Source: CAD feature listing. Evaluate the final solid. Frame: model axes, mm. Face numbers are marked on the shaded views. A direction names the side the tool comes from. Give positions to 0.01 mm unless a question says otherwise; leave off trailing zeros. Loops run counter-clockwise (first coordinate to the right, second up) from the corner with the lowest first, then second, coordinate; pieces in that order, holes last. Notation, with made-up numbers: (60, 32) -> (100, 32) arc R8 cw to (100, 46) -> close; hole circle Ø5 at (-27, -0.75). An arc over 180 degrees is marked (long way). Answer as a JSON object with one key per item and string values. Group by question number.
from build123d import *

# Parameters (mm, degrees)
SKETCH1_W           = 40
SKETCH1_H           = 40
SKETCH1_R           = 2
BOSS_EXTRUDE1_DEPTH = 1
SKETCH2_W           = 40
SKETCH2_H           = 1
BOSS_EXTRUDE2_DEPTH = 46
CUT_EXTRUDE1_DEPTH  = 46


with BuildPart() as part:
    # Sketch1 → Boss-Extrude1 (new body)
    with BuildSketch(Plane(origin=(0, 0, 0), x_dir=(1, 0, 0), z_dir=(0, 1, 0))):
        Rectangle(SKETCH1_W, SKETCH1_H)
        with Locations(Location((-15, -12, 0), (0, 0, 270))):
            Circle(SKETCH1_R, mode=Mode.SUBTRACT)
        with Locations(Location((15, -12, 0), (0, 0, 270))):
            Circle(SKETCH1_R, mode=Mode.SUBTRACT)
        with Locations(Location((15, 12, 0), (0, 0, 270))):
            Circle(SKETCH1_R, mode=Mode.SUBTRACT)
        with Locations(Location((-15, 12, 0), (0, 0, 270))):
            Circle(SKETCH1_R, mode=Mode.SUBTRACT)
    extrude(amount=BOSS_EXTRUDE1_DEPTH)

    # Sketch2 → Boss-Extrude2 (add)
    with BuildSketch(Plane(origin=(0, 1, 0), x_dir=(1, 0, 0), z_dir=(0, 1, 0))):
        with Locations((0, 19.5)):
            Rectangle(SKETCH2_W, SKETCH2_H)
    extrude(amount=BOSS_EXTRUDE2_DEPTH)

    # Sketch3 → Cut-Extrude1 (cut)
    with BuildSketch(Plane.XY.offset(-19)):
        with BuildLine():
            Line((6, 19), (6, 35))
            ThreePointArc((6, 35), (0, 41), (-6, 35))
            Line((-6, 35), (-6, 19))
            ThreePointArc((-6, 19), (0, 13), (6, 19))
        make_face()
        with BuildLine():
            Line((-20, 47), (-20, 27))
            ThreePointArc((-20, 27), (-14.142135559, 41.142135688), (1.83e-07, 47))
            Line((1.83e-07, 47), (-20, 47))
        make_face()
        with BuildLine():
            ThreePointArc((1.83e-07, 47), (14.142135688, 41.142135559), (20, 27))
            Line((20, 27), (20, 47))
            Line((20, 47), (1.83e-07, 47))
        make_face()
    extrude(amount=-CUT_EXTRUDE1_DEPTH, mode=Mode.SUBTRACT)


solid = part.part
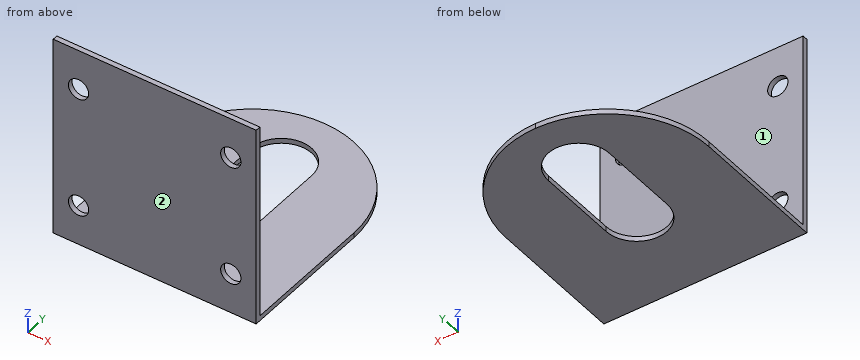
(1) Section query B-B on z = 12. Return the cut outline in (x, y), plus the area to 3 significant figures.
(2) Section query C-C on x = 15. Return the cut outline in (y, z), plus the area to 3 significant figures.
(3) First-contact query: pin 1 (3 mm diameter, centred on x = -15, z = 12, fed in from +Y); pin 2 (2 mm diameter, centred on x = -3, y = 7.5, fed in from +Z); pin 3 (19.5 mm diameter, centred on x = 0, z = -6, fed in from +Y); pin 4 (0.8 mm diameter, centred on y = 30, z = -19.5, fed in from +X). Flat tips, straight axial feed; report the tip coordinate or a pass-through.
(4) Section query A-A on y = 22. Return the cut outline in (x, z).
(5) Section query D-D on z = -6. Return the cut outline in (x, y).
(6) Access query for the marked faces 1 and 2. Directions: +Z, -Z, +X, -X, +Y, -Y. A direction counts if a zero-diameter tool reaches every point of the face in a straight line with its end or side. Return the directions, or none.
(7) Material intervals for line 1 (X direction, y = 0.5, z = 12); line 2 (Y direction, x = 6.5, z = 18); line 3 (Z direction, x = -2.5, y = 11.5), sorted ascending. Write a range as from..to.
Result:
{
 "1": {"outline": "(-20, 0) -> (-17, 0) -> (-17, 1) -> (-20, 1) -> close; (-13, 0) -> (13, 0) -> (13, 1) -> (-13, 1) -> close; (17, 0) -> (20, 0) -> (20, 1) -> (17, 1) -> close", "area": "32.0 mm²"},
 "2": {"outline": "(0, -20) -> (40.23, -20) -> (40.23, -19) -> (1, -19) -> (1, -14) -> (0, -14) -> close; (0, -10) -> (1, -10) -> (1, 10) -> (0, 10) -> close; (0, 14) -> (1, 14) -> (1, 20) -> (0, 20) -> close", "area": "71.2 mm²"},
 "3": {"pin 1": "through", "pin 2": "z = -19", "pin 3": "y = 1", "pin 4": "x = 19.83"},
 "4": {"outline": "(-20, -20) -> (-6, -20) -> (-6, -19) -> (-20, -19) -> close; (6, -20) -> (20, -20) -> (20, -19) -> (6, -19) -> close"},
 "5": {"outline": "(-20, 0) -> (20, 0) -> (20, 1) -> (-20, 1) -> close"},
 "6": {"face 1": "+Z, +X, -X, +Y", "face 2": "+Z, -Z, +X, -X, -Y"},
 "7": {"line 1": "-20..-17, -13..13, 17..20", "line 2": "0..1", "line 3": "-20..-19"}
}
